Part model, mm, in its own coordinate system. A direction names the side the tool comes from. Round coordinates to 2 decimals unless told otherwise and drop trailing zeros. Loops run counter-clockwise (first coordinate to the right, second up) from the corner with the lowest first, then second, coordinate; pieces in that order, holes last. Notation, with made-up numbers: (-2, 87.25) - (53, 87.25) arc R25 ccw to (53, 126.25) - close; hole circle Ø8 at (89.5, 67.25). An arc over 180 degrees is marked (long way). Put each result on its own line as item: value.
from build123d import *

# Parameters (mm, degrees)
BOSS_EXTRUDE1_DEPTH = 20
FILLET1_R           = 2
SKETCH4_R           = 11
CUT_EXTRUDE2_DEPTH  = 6.35
SKETCH5_OUTSIDE_W   = 143.42
SKETCH5_OUTSIDE_H   = 293.42
CUT_EXTRUDE3_DEPTH  = 10
SKETCH7_R           = 2
CUT_EXTRUDE4_DEPTH  = 11
SKETCH9_W           = 20
SKETCH9_H           = 50.969748303
CUT_EXTRUDE6_DEPTH  = 21
SKETCH10_W          = 35
SKETCH10_H          = 18
BOSS_EXTRUDE2_DEPTH = 43.9


with BuildPart() as part:
    # Sketch1 → Boss-Extrude1 (new body)
    with BuildSketch(Plane(origin=(0, 0, 0), x_dir=(1, 0, 0), z_dir=(0, 1, 0))):
        with BuildLine():
            Line((0, 0), (0, 150))
            ThreePointArc((0, 150), (-45, 195), (-90, 150))
            Line((-90, 150), (-90, 0))
            ThreePointArc((-90, 0), (-45, -45), (0, 0))
        make_face()
    extrude(amount=-BOSS_EXTRUDE1_DEPTH)

    # Fillet1
    fillet1_edges = [part.edges().sort_by_distance(p)[0] for p in [
        (-45, -20, -195),
        (-90, -20, -75),
        (-45, -20, 45),
        (-90, 0, -75),
        (-45, 0, -195),
        (0, 0, -75),
        (-45, 0, 45),
        (0, -20, -75),
    ]]
    fillet(fillet1_edges, radius=FILLET1_R)

    # Sketch4 → Cut-Extrude2 (cut)
    with BuildSketch(Plane.XZ.offset(20)):
        with Locations((-45.5, -150)):
            Circle(SKETCH4_R)
    extrude(amount=-CUT_EXTRUDE2_DEPTH, mode=Mode.SUBTRACT)

    # Sketch5 outside → Cut-Extrude3 (cut)
    with BuildSketch(Plane(origin=(0, 0, 0), x_dir=(1, 0, 0), z_dir=(0, 1, 0))):
        with Locations((-45, 75)):
            Rectangle(SKETCH5_OUTSIDE_W, SKETCH5_OUTSIDE_H)
        with BuildLine():
            Line((-78, 0), (-78, 150))
            ThreePointArc((-78, 150), (-45, 183), (-12, 150))
            Line((-12, 150), (-12, 0))
            ThreePointArc((-12, 0), (-45, -33), (-78, 0))
        make_face(mode=Mode.SUBTRACT)
    extrude(amount=-CUT_EXTRUDE3_DEPTH, mode=Mode.SUBTRACT)

    # Sketch7 → Cut-Extrude4 (cut, through all)
    with BuildSketch(Plane(origin=(0, -10, 0), x_dir=(1, 0, 0), z_dir=(0, 1, 0))):
        with Locations((-6, 75)):
            Circle(SKETCH7_R)
        with Locations((-6, 115)):
            Circle(SKETCH7_R)
        with Locations((-6, 155)):
            Circle(SKETCH7_R)
        with Locations((-6, 35)):
            Circle(SKETCH7_R)
        with Locations((-6, -5)):
            Circle(SKETCH7_R)
        with Locations((-84, -5)):
            Circle(SKETCH7_R)
        with Locations((-84, 35)):
            Circle(SKETCH7_R)
        with Locations((-84, 75)):
            Circle(SKETCH7_R)
        with Locations((-84, 115)):
            Circle(SKETCH7_R)
        with Locations((-84, 155)):
            Circle(SKETCH7_R)
    extrude(amount=-CUT_EXTRUDE4_DEPTH, mode=Mode.SUBTRACT)

    # Sketch9 → Cut-Extrude6 (cut, through all)
    with BuildSketch(Plane(origin=(0, 0, 0), x_dir=(1, 0, 0), z_dir=(0, 1, 0))):
        with Locations((-45, -25.484874152)):
            Rectangle(SKETCH9_W, SKETCH9_H)
    extrude(amount=-CUT_EXTRUDE6_DEPTH, mode=Mode.SUBTRACT)

    # Sketch10 → Boss-Extrude2 (add)
    with BuildSketch(Plane.XY):
        with Locations((-17.5, -9)):
            Rectangle(SKETCH10_W, SKETCH10_H)
    extrude(amount=BOSS_EXTRUDE2_DEPTH)


solid = part.part
1. Pin check, flat tips, straight feed: P1, Ø2, axis at x = -64.5, y = -12, coming from the +Z side; P2, Ø3, axis at y = -8, z = -64.5, coming from the +X side; P3, Ø2.5, axis at x = -6, z = -155, coming from the -Y side; P4, Ø3, axis at y = -5, z = -72.5, coming from the -X side. Stop position of each tip, or through.
A:
P1: stops at z = 41.02
P2: stops at x = -12
P3: passes through
P4: stops at x = -78
2. Two-plate mould, pull along X, no slides. Class faces 5 (the flat face through (-90, -14, -76)), 6 (the flat face through (-55, -10, 17)), 7 (the flat face through (-46, -20, -77)), 8 (the flat face through (-35, -10, 22)): pulls with the +X half, pulls with the -X half, needs draft (parallel to the pull), parting line crosses it, or undercut.
A:
face 5: pulls with the -X half
face 6: undercut
face 7: needs draft
face 8: undercut
3. Band-saw the part on A-A (z = -42). List the corners of the cut face in (x, y), plus the area to 3 significant figures.
A:
outline: (-90, -18) arc R2 ccw to (-88, -20) - (-2, -20) arc R2 ccw to (0, -18) - (0, -10) - (-12, -10) - (-12, 0) - (-78, 0) - (-78, -10) - (-90, -10) - close
area: 1,560 mm²
4. Tool access for faces 1 (the cylindrical face through (-45.73, -4.93, -182.99)), 2 (the flat face through (-6, -5, 0)), 3 (the flat face through (-46, -13.65, -150)), 4 (the flat face through (-9, -18, 35)): list every direction of +Z, -Z, +X, -X, +Y, -Y with a clear straight run to the whole face (end or side of a thin tool).
A:
face 1: -Z, +Y
face 2: -Z, +X, +Y
face 3: -Y
face 4: +Z, +X, -Y
5. Probe line 1 along X through (y, z) = (-14.75, -115); line 2 along Z through (x, y) = (-6, -14.5); line 3 along X through (y, z) = (-13.25, -155). List the from-to ranges inside material, lowest first. Write a range as [from, to].
A:
line 1: x = [-90, -86], [-82, -8], [-4, 0]
line 2: z = [-172.45, -157], [-153, -117], [-113, -77], [-73, -37], [-33, 43.9]
line 3: x = [-89.72, -86], [-82, -8], [-4, -0.28]
